Print and shaded views of the part. All mm, measured from the part's lowest x, y and z. Give positions to 0.01 mm unless a question says otherwise; leave off trailing zeros. Write each loop counter-clockwise with the first axis right and the second up, starting at its lowest first coordinate (ties: lowest second). Pieces come first, ordered by that corner, then holes. Notation, with made-up numbers: (84, -39) -> (88, -39) arc R29 ccw to (88, -1) -> close; hole circle Ø7 at (57.5, 32.25). An arc over 180 degrees is marked (long way). Put each result on its own line as item: value.
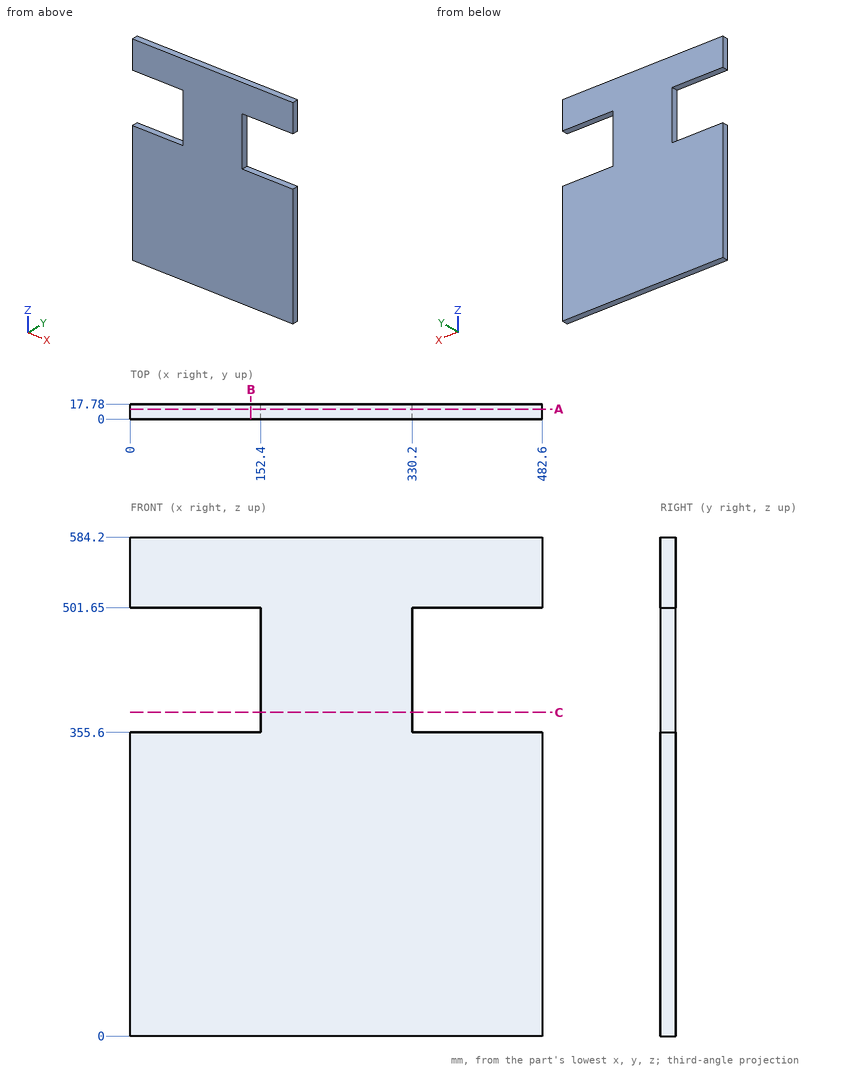
1) Wall check: L1, parallel to Z at x = 404, y = 15.75; L2, parallel to X at y = 4, z = 460.5. Give the ranges that are in metal, low to high.
Filled sheet:
L1: 0 to 355.6, 501.65 to 584.2
L2: 152.4 to 330.2
2) Slice it at A-A (y = 11.75). Write the cut outline in (x, z).
Filled sheet:
outline: (0, 0) -> (482.6, 0) -> (482.6, 355.6) -> (330.2, 355.6) -> (330.2, 501.65) -> (482.6, 501.65) -> (482.6, 584.2) -> (0, 584.2) -> (0, 501.65) -> (152.4, 501.65) -> (152.4, 355.6) -> (0, 355.6) -> close
3) Slice it at B-B (x = 141). Write the cut outline in (y, z), plus the area to 3 significant figures.
Filled sheet:
outline: (0, 0) -> (17.78, 0) -> (17.78, 355.6) -> (0, 355.6) -> close; (0, 501.65) -> (17.78, 501.65) -> (17.78, 584.2) -> (0, 584.2) -> close
area: 7,790 mm2
4) Pin check, flat tip, straight feed: pin 1 (5.5 mm diameter, centred on y = 11, z = 452, fed in from +X). Stop position of the tip, or through.
Filled sheet:
pin 1: x = 330.2
5) Slice it at C-C (z = 379). Write the cut outline in (x, y), plus the area to 3 significant figures.
Filled sheet:
outline: (152.4, 0) -> (330.2, 0) -> (330.2, 17.78) -> (152.4, 17.78) -> close
area: 3,160 mm2
